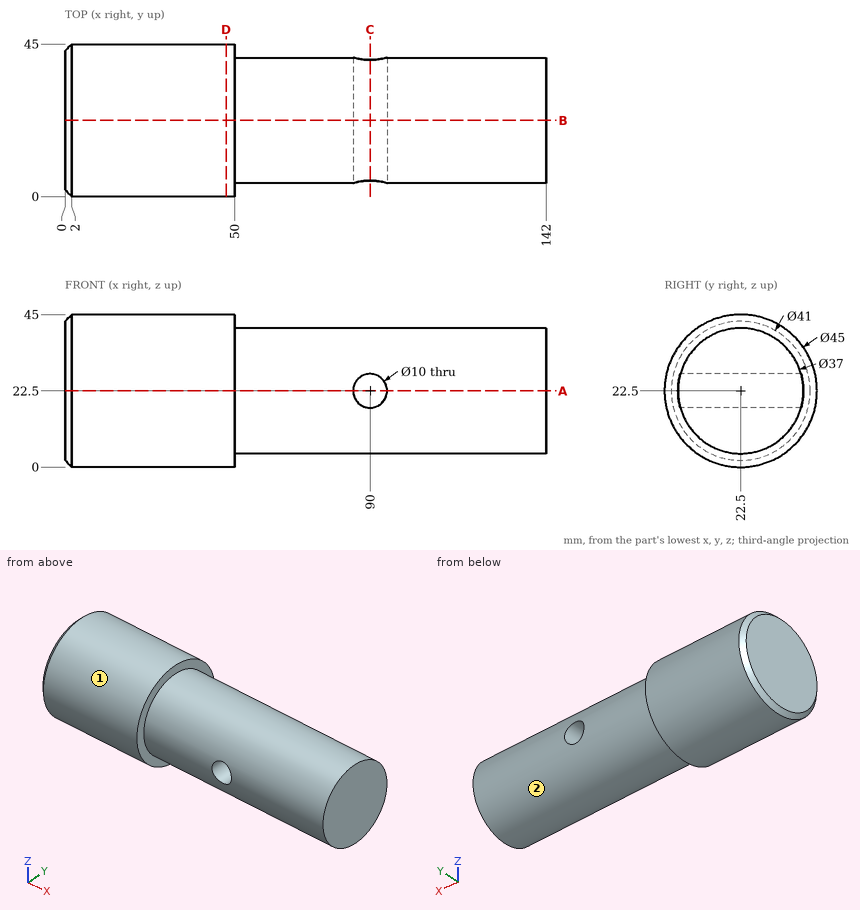
Here's the drawing with two shaded views (mm, measured from the low corner). I have some questions. A direction names the side the tool comes from. Coordinates: 2 decimals unless noted, no trailing zeros. Write each loop counter-clockwise with the first axis right and the second up, starting at its lowest first coordinate (ties: lowest second). Pieces come first, ordered by that corner, then holes. Notation, with made-up numbers: (81, -15) -> (137, -15) arc R27 ccw to (137, 20) -> close; hole circle Ø1 at (45, 54.25). An arc over 180 degrees is marked (long way). Write item = value, one per line. Start each with the question number.
(1) Will these pins go through, and if not, where does the flat tip stop? pin 1 (4 mm diameter, centred on x = 59, z = 37, fed in from +Y); pin 2 (12 mm diameter, centred on x = 17, y = 10, fed in from -Z); pin 3 (1 mm diameter, centred on x = 49, y = 11, fed in from +Z).
(2) I want a section at A-A (z = 22.5). Please give me the cut outline in (x, y).
(3) I want a section at C-C (x = 90). Please give me the cut outline in (y, z), plus the area to 3 significant figures.
(4) I want a section at B-B (y = 22.5). Please give me the cut outline in (x, z), plus the area to 3 significant figures.
(5) I need wall thicknesses on line 1 (X direction, y = 27.5, z = 22.5); line 2 (Z direction, x = 90, y = 23.5); line 3 (Z direction, x = 90, y = 25). Which ranges of each line are inside material? Lowest first, please. Write a range as [from, to].
(6) Which directions (+Z, -Z, +X, -X, +Y, -Y) give clear straight access to the entire face, cutting with the end or side of a thin tool? Please do the marked faces 1 and 2.
(7) I want a section at D-D (x = 47.5). Please give me the cut outline in (y, z).
Result set:
q1.pin_1 = 36.14
q1.pin_2 = 0.96
q1.pin_3 = 42.13
q2.outline = (0, 2) -> (2, 0) -> (50, 0) -> (50, 4) -> (85, 4) -> (85, 41) -> (50, 41) -> (50, 45) -> (2, 45) -> (0, 43) -> close; (95, 4) -> (142, 4) -> (142, 41) -> (95, 41) -> close
q3.outline = (4.69, 17.5) arc R18.5 ccw to (40.31, 17.5) -> close; (4.69, 27.5) -> (40.31, 27.5) arc R18.5 ccw to start
q3.area = 710 mm2
q4.outline = (0, 2) -> (2, 0) -> (50, 0) -> (50, 4) -> (142, 4) -> (142, 41) -> (50, 41) -> (50, 45) -> (2, 45) -> (0, 43) -> close; hole circle Ø10 at (90, 22.5)
q4.area = 5,570 mm2
q5.line_1 = [0, 85], [95, 142]
q5.line_2 = [4.03, 17.5], [27.5, 40.97]
q5.line_3 = [4.17, 17.5], [27.5, 40.83]
q6.face_1 = +X, -X
q6.face_2 = +X
q7.outline = circle Ø45 at (22.5, 22.5)
